from build123d import *

# Parameters (mm, degrees)
F0_W     = 109.020278
F0_H     = 50
F1_DEPTH = 45
F3_DEPTH = 207
F4_W     = 72.165563
F4_H     = 35
F5_DEPTH = 228


with BuildPart() as f1:
    # F0 (on Right) → F1 (new body)
    with BuildSketch(Plane.YZ):
        with Locations((2.837837, -9.1723)):
            Rectangle(F0_W, F0_H)
    extrude(amount=F1_DEPTH)

    # F2 (on face) → F3 (cut)
    with BuildSketch(Plane.YZ.offset(45)):
        Polygon((-51.672302, 0), (-43.100026, 15.8277), (-51.672302, 15.8277), align=None)
    extrude(amount=-F3_DEPTH, mode=Mode.SUBTRACT)

    # F4 (on face) → F5 (cut)
    with BuildSketch(Plane.YZ.offset(45)):
        with Locations((2.14697, -1.6723)):
            Rectangle(F4_W, F4_H)
    extrude(amount=-F5_DEPTH, mode=Mode.SUBTRACT)


solid = f1.part
Design review of the part built by this model. Coordinates are the model's own, in mm. A direction names the side the tool comes from. Give positions to 0.01 mm unless a question says otherwise; leave off trailing zeros. Order: outer loops, then holes, each group sorted by start corner. A loop starts at its lowest first (then second) coordinate and runs counter-clockwise, first axis right, second up.
1. For pin 1 Ø13.5 at (x, y) = (27.5, -15) entering from +Z, flat-tipped, find the tip position at first contact; note if it passes through.
Solution:
pin 1: stops at z = -19.17
2. Add section C-C, the plane z = 8.5. State the section outline as (x, y) points.
Solution:
outline: (0, -47.07) - (45, -47.07) - (45, -33.94) - (0, -33.94) - close; (0, 38.23) - (45, 38.23) - (45, 57.35) - (0, 57.35) - close
3. Add section D-D, the plane y = -11.5. State the section outline as (x, z) points.
Solution:
outline: (0, -34.17) - (45, -34.17) - (45, -19.17) - (0, -19.17) - close
4. Mouldability with a two-part tool opening along Y and no side actions: class faces 3 (the flat face through (22.82, -47.45, 7.8)), 4 (the flat face through (23, 38.23, -2)), 5 (the flat face through (0, 2, -20)) as +Y half, -Y half, draft (parallel to the pull), parting line (faces both ways), or undercut.
Solution:
face 3: -Y half
face 4: undercut
face 5: draft
5. To check wall thickness, follow L1, parallel to Y at x = 11.5, z = -9; L2, parallel to Z at x = 37, y = -16.5; L3, parallel to Y at x = 40.5, z = 12. State the ranges of each line that lie inside material, in increasing order.
Solution:
L1: y = -51.67 to -33.94, 38.23 to 57.35
L2: z = -34.17 to -19.17
L3: y = -45.17 to -33.94, 38.23 to 57.35
6. Add section B-B, the plane x = 6.5. State the section outline as (y, z) points, then the cut area to 3 significant figures.
Solution:
outline: (-51.67, -34.17) - (57.35, -34.17) - (57.35, 15.83) - (38.23, 15.83) - (38.23, -19.17) - (-33.94, -19.17) - (-33.94, 15.83) - (-43.1, 15.83) - (-51.67, 0) - close
area: 2,860 mm2
7. Add section A-A, the plane z = -4. State the section outline as (x, y) points, then the cut area to 3 significant figures.
Solution:
outline: (0, -51.67) - (45, -51.67) - (45, -33.94) - (0, -33.94) - close; (0, 38.23) - (45, 38.23) - (45, 57.35) - (0, 57.35) - close
area: 1,660 mm2
8. Tool access review of faces 1 (the flat face through (23, -33.936, -2)), 2 (the flat face through (22, 57.348, -10)): name each direction out of +Z, -Z, +X, -X, +Y, -Y from which nothing blocks a thin tool from reaching the whole face with its end or side.
Solution:
face 1: +Z, +X, -X
face 2: +Z, -Z, +X, -X, +Y
